from build123d import *
from build123d.topology import SkipClean

# Parameters (mm, degrees)
BOSS_EXTRUDE1_DEPTH = 2
BOSS_EXTRUDE2_START = 4.5
SKETCH2_R           = 6
SKETCH2_R_2         = 3
BOSS_EXTRUDE2_DEPTH = 4.5
CHAMFER1_SIZE       = 1
BOSS_EXTRUDE3_START = 5
SKETCH3_R           = 1
BOSS_EXTRUDE3_DEPTH = 5
BOSS_EXTRUDE4_START = 15
SKETCH4_R           = 3
SKETCH4_R_2         = 1.5
BOSS_EXTRUDE4_DEPTH = 15
SKETCH5_R           = 1.5
BOSS_EXTRUDE5_DEPTH = 3
CUT_EXTRUDE1_DEPTH  = 1


with BuildPart() as part:
    # Sketch1 → Boss-Extrude1 (new body)
    with BuildSketch(Plane.XY):
        with BuildLine():
            Line((-5.196152423, 3), (-19.603847577, 3))
            ThreePointArc((-19.603847577, 3), (-22.176137566, 5.39586378), (-25.649056604, 5.939621443))
            Line((-25.649056604, 5.939621443), (-46.424528302, 2.969810721))
            ThreePointArc((-46.424528302, 2.969810721), (-49, 0), (-46.424528302, -2.969810721))
            Line((-46.424528302, -2.969810721), (-25.649056604, -5.939621443))
            ThreePointArc((-25.649056604, -5.939621443), (-22.176137566, -5.39586378), (-19.603847577, -3))
            Line((-19.603847577, -3), (-5.196152423, -3))
            ThreePointArc((-5.196152423, -3), (-4.560521825, -3.898928146), (-3.771341235, -4.666581756))
            Line((-3.771341235, -4.666581756), (15.614329382, -20.333290878))
            ThreePointArc((15.614329382, -20.333290878), (17.066851522, -20.968565714), (18.640337336, -20.774820852))
            Line((18.640337336, -20.774820852), (33.240337336, -14.774820852))
            ThreePointArc((33.240337336, -14.774820852), (34.592088683, -13.670177833), (35.1, -12))
            Line((35.1, -12), (35.1, 12))
            ThreePointArc((35.1, 12), (34.592088683, 13.670177833), (33.240337336, 14.774820852))
            Line((33.240337336, 14.774820852), (18.640337336, 20.774820852))
            ThreePointArc((18.640337336, 20.774820852), (17.066851522, 20.968565714), (15.614329382, 20.333290878))
            Line((15.614329382, 20.333290878), (-3.771341235, 4.666581756))
            ThreePointArc((-3.771341235, 4.666581756), (-4.560521825, 3.898928146), (-5.196152423, 3))
        make_face()
        with BuildLine():
            Line((7.677811186, 1.954226556), (16.302661255, 12))
            Line((16.302661255, 12), (29.1, 12))
            Line((29.1, 12), (29.1, -12))
            Line((29.1, -12), (16.302661255, -12))
            Line((16.302661255, -12), (7.677811186, -1.954226556))
            ThreePointArc((7.677811186, -1.954226556), (6.953991883, 0), (7.677811186, 1.954226556))
        make_face(mode=Mode.SUBTRACT)
    extrude(amount=-BOSS_EXTRUDE1_DEPTH)

    # Sketch2 → Boss-Extrude2 (add)
    # profile 1 of 2: a face of its own
    with BuildSketch(Plane.XY.offset(BOSS_EXTRUDE2_START)):
        with Locations((-24.8, 0)):
            Circle(SKETCH2_R)
        with Locations((-24.8, 0)):
            Circle(SKETCH2_R_2, mode=Mode.SUBTRACT)
    # profile 2 of 2: a face of its own
    with BuildSketch(Plane.XY.offset(BOSS_EXTRUDE2_START)):
        Circle(SKETCH2_R)
        Circle(SKETCH2_R_2, mode=Mode.SUBTRACT)
    extrude(amount=-BOSS_EXTRUDE2_DEPTH)

    # Chamfer1
    chamfer1_edges = [part.edges().sort_by_distance(p)[0] for p in [
        (-30.8, 0, 4.5),
        (-6, 0, 4.5),
    ]]
    chamfer(chamfer1_edges, length=CHAMFER1_SIZE)

    # Sketch3 → Boss-Extrude3 (add)
    # profile 1 of 3: a face of its own
    with SkipClean():  # the faces are left unmerged after this step: merging them gives an invalid solid
        with BuildSketch(Plane.XY.offset(BOSS_EXTRUDE3_START)):
            with BuildLine():
                Line((-44, -2.236067977), (-44, 2.236067977))
                ThreePointArc((-44, 2.236067977), (-49, 0), (-44, -2.236067977))
            make_face()
            with Locations((-46, 0)):
                Circle(SKETCH3_R, mode=Mode.SUBTRACT)
        # profile 2 of 3: a face of its own
        with BuildSketch(Plane.XY.offset(BOSS_EXTRUDE3_START)):
            with BuildLine():
                Line((14.714743135, -16.885395049), (18.917176291, -15.355834468))
                ThreePointArc((18.917176291, -15.355834468), (18.52606043, -20.819077862), (14.714743135, -16.885395049))
            make_face()
            with Locations((17.5, -18)):
                Circle(SKETCH3_R, mode=Mode.SUBTRACT)
        # profile 3 of 3: a face of its own
        with BuildSketch(Plane.XY.offset(BOSS_EXTRUDE3_START)):
            with BuildLine():
                Line((14.714743135, 16.885395049), (18.917176291, 15.355834468))
                ThreePointArc((18.917176291, 15.355834468), (18.52606043, 20.819077862), (14.714743135, 16.885395049))
            make_face()
            with Locations((17.5, 18)):
                Circle(SKETCH3_R, mode=Mode.SUBTRACT)
        extrude(amount=-BOSS_EXTRUDE3_DEPTH)

    # Sketch4 → Boss-Extrude4 (add)
    # profile 1 of 2: a face of its own
    with SkipClean():  # the faces are left unmerged after this step: merging them gives an invalid solid
        with BuildSketch(Plane.XY.offset(BOSS_EXTRUDE4_START)):
            with Locations((32.1, -12)):
                Circle(SKETCH4_R)
            with Locations((32.1, -12)):
                Circle(SKETCH4_R_2, mode=Mode.SUBTRACT)
        # profile 2 of 2: a face of its own
        with BuildSketch(Plane.XY.offset(BOSS_EXTRUDE4_START)):
            with Locations((32.1, 12)):
                Circle(SKETCH4_R)
            with Locations((32.1, 12)):
                Circle(SKETCH4_R_2, mode=Mode.SUBTRACT)
        extrude(amount=-BOSS_EXTRUDE4_DEPTH)

    # Sketch5 → Boss-Extrude5 (add)
    with BuildSketch(Plane.XY.offset(15)):
        with BuildLine():
            Line((29.446176569, -13.399007218), (26.6, -8))
            Line((26.6, -8), (26.6, 8))
            Line((26.6, 8), (29.446176569, 13.399007218))
            ThreePointArc((29.446176569, 13.399007218), (32.1, 15), (34.753823431, 13.399007218))
            Line((34.753823431, 13.399007218), (37.6, 8))
            Line((37.6, 8), (37.6, -8))
            Line((37.6, -8), (34.753823431, -13.399007218))
            ThreePointArc((34.753823431, -13.399007218), (32.1, -15), (29.446176569, -13.399007218))
        make_face()
        with Locations((32.1, -12)):
            Circle(SKETCH5_R, mode=Mode.SUBTRACT)
        with Locations((32.1, 12)):
            Circle(SKETCH5_R, mode=Mode.SUBTRACT)
    extrude(amount=-BOSS_EXTRUDE5_DEPTH)

    # Sketch6 → Cut-Extrude1 (cut)
    with BuildSketch(Plane.XY.offset(15)):
        with BuildLine():
            Line((29.446176569, 13.399007218), (26.6, 8))
            Line((26.6, 8), (26.6, 6))
            Line((26.6, 6), (37.6, 6))
            Line((37.6, 6), (37.6, 8))
            Line((37.6, 8), (34.753823431, 13.399007218))
            ThreePointArc((34.753823431, 13.399007218), (32.1, 9), (29.446176569, 13.399007218))
        make_face()
        with BuildLine():
            Line((26.6, -8), (29.446176569, -13.399007218))
            ThreePointArc((29.446176569, -13.399007218), (32.1, -9), (34.753823431, -13.399007218))
            Line((34.753823431, -13.399007218), (37.6, -8))
            Line((37.6, -8), (37.6, -6))
            Line((37.6, -6), (26.6, -6))
            Line((26.6, -6), (26.6, -8))
        make_face()
    extrude(amount=-CUT_EXTRUDE1_DEPTH, mode=Mode.SUBTRACT)


solid = part.part
Work out the finished part from the listing and answer in its coordinate system (mm). A direction names the side the tool comes from. Coordinates: 2 decimals unless noted, no trailing zeros. Loops run counter-clockwise (first coordinate to the right, second up) from the corner with the lowest first, then second, coordinate; pieces in that order, holes last. Notation, with made-up numbers: M 79,68 L 122,68 A15 cw 122,94 Z; hole C 85,11.25 d4. An arc over 180 degrees is marked long. Answer in a Markdown table with one row per item. Add a question column.
1. The mould has two halves that part along X. Classify faces 1 (the flat face through (37.6, 0, 14)), 2 (the flat face through (33.4, -13.3, 15)), 3 (the cylindrical face through (6.954, -0.03, -0.986)), 4 (the flat face through (28.003, 10.662, 13.014)): pulls with the +X half, pulls with the -X half, needs draft (parallel to the pull), parting line crosses it, or undercut.
2. Consider L1, parallel to Y at x = 32.1, z = 13.45; L2, parallel to Y at x = -24.8, z = 3.3; L3, parallel to Z at x = 32, y = -4. Determine where each line is inside the solid, lowest interval first.
3. Find section A-A, the plane z = 2. State how many separate pieces and enclosed holes the cut face has, then the cut area to 3 significant figures.
4. Flat-ended cylindrical pins translate along their axes: P1, Ø6.5, axis at x = -24, y = -0.5, coming from the +Z side; P2, Ø1, axis at y = -1.5, z = -1, coming from the -X side; P3, Ø10, axis at y = -6, z = 4, coming from the +X side. Find the tip coordinate at first contact, or state that the pin passes through.
5. A tool of negligible diameter and unlimited length cuts with its end or side. For faces 5 (the flat face through (29.1, 0, -1)), 6 (the flat face through (17.5, -19.4, 5)), 7 (the flat face through (-0.1, -3.3, 4.5)), 8 (the cylindrical face through (-3, 0, 2)), 9 (the flat face through (-36.182, -4.434, -0.986)), from which of +Z, -Z, +X, -X, +Y, -Y can it reach the whole face along a straight path? Write none if from no direction.
6. Find section C-C, the plane x = 17.5. Write down the section's boundary in (y, z).
7. Find section B-B, the plane z = 9.5. Write down the section's boundary in (x, y), then the cut area to 3 significant figures.
Reported:
| question | item | result |
|---|---|---|
| 1 | face 1 | pulls with the +X half |
| 1 | face 2 | needs draft |
| 1 | face 3 | undercut |
| 1 | face 4 | pulls with the -X half |
| 2 | L1 | y = -15 to -13.5, -10.5 to 10.5, 13.5 to 15 |
| 2 | L2 | y = -6 to -3, 3 to 6 |
| 2 | L3 | z = -2 to 0, 12 to 15 |
| 3 | separate pieces | 7 |
| 3 | enclosed holes | 7 |
| 3 | area | 278 mm^2 |
| 4 | P1 | stops at z = 4.5 |
| 4 | P2 | stops at x = -48.83 |
| 4 | P3 | stops at x = 35.1 |
| 5 | face 5 | -Z |
| 5 | face 6 | +Z, +X, -X, +Y, -Y |
| 5 | face 7 | +Z, +X, +Y, -Y |
| 5 | face 8 | +Z |
| 5 | face 9 | +Z, -Z, -X, -Y |
| 6 | outline | M -21,-2 L -12,-2 L -12,0 L -15.87,0 L -15.87,5 L -17,5 L -17,0 L -19,0 L -19,5 L -21,5 Z; M 12,-2 L 21,-2 L 21,5 L 19,5 L 19,0 L 17,0 L 17,5 L 15.87,5 L 15.87,0 L 12,0 Z |
| 7 | outline | C 32.1,-12 d6; C 32.1,12 d6; hole C 32.1,-12 d3; hole C 32.1,12 d3 |
| 7 | area | 42.4 mm^2 |
